Autodesk Inventor part; units mm, degrees
ref_plane "YZ Plane" through (0, 0, 0) normal (1, 0, 0) x (0, 1, 0)
ref_plane "XZ Plane" through (0, 0, 0) normal (0, 1, 0) x (-1, 0, 0)
ref_plane "XY Plane" through (0, 0, 0) normal (0, 0, 1) x (1, 0, 0)
sketch "Sketch1" plane through (0, 0, 0) normal (0, 0, 1) x (1, 0, 0)
  line L0 (20.2828, 57.747) -> (62.7008, 57.747)
  line L1 (62.7008, 57.747) -> (62.7008, 15.329)
  line L2 (62.7008, 15.329) -> (20.2828, 15.329)
  line L3 (20.2828, 15.329) -> (20.2828, 57.747)
  dimension "d0" = 42.418
  dimension "d1" = 42.418
extrude "Extrusion1" add sketch "Sketch1" along normal blind 48.006
sketch "Sketch2" plane through (0, 0, 48.006) normal (0, 0, 1) x (1, 0, 0)
  line L0 (20.2828, 57.747) -> (62.7008, 57.747)
  line L1 (20.2828, 15.329) -> (20.2828, 57.747)
  circle A0 centre (25.9978, 52.032) radius 1.5
  dimension "d4" = 3
  dimension "d5" = 5.715
  dimension "d6" = 5.715
hole "Hole1" at (25.9978, 52.032, 48.006) direction (0, 0, -1) diameter 2.4638 depth 4.5 tip angle 118
pattern_linear "Rectangular Pattern1" count 2 spacing 30.988 along (1, 0, 0) count 2 spacing 30.988 along (0, -1, 0) of "Hole1"
sketch "Sketch3" plane through (0, 0, 48.006) normal (0, 0, 1) x (1, 0, 0)
  circle A0 centre (41.4918, 36.538) radius 11.049
  dimension "d20" = 22.098
extrude "Extrusion2" add sketch "Sketch3" along normal blind 2
sketch "Sketch4" plane through (41.4918, 36.538, 50.006) normal (0, 0, 1) x (1, 0, 0)
  circle A0 centre (0, 0) radius 11.049
  circle A1 centre (0, 0) radius 2.5
  dimension "d23" = 5
extrude "Extrusion3" add sketch "Sketch4" along normal blind 22 contours A1
chamfer "Chamfer1" distance 7 angle 45 4 edges at (62.7008, 57.747, 24.003) (20.2828, 57.747, 24.003) (20.2828, 15.329, 24.003) (62.7008, 15.329, 24.003)
sketch "Sketch5" plane through (0, 0, 0) normal (0, 0, -1) x (-1, 0, 0)
  line L0 (-27.2828, 57.747) -> (-55.7008, 57.747)
  line L1 (-62.7008, 50.747) -> (-62.7008, 22.329)
  circle A0 centre (-41.4918, 36.538) radius 2.5
  dimension "d29" = 5
  dimension "d30" = 21.209
  dimension "d31" = 21.209
extrude "Extrusion4" add sketch "Sketch5" along normal blind 10
properties part number "SM-E01" material "Aluminum-6061"
Input: part model. Units: mm. Frame: model coordinates. A direction names the side the tool comes from. Coordinates: 2 decimals unless noted, no trailing zeros. Loops run counter-clockwise (first coordinate to the right, second up) from the corner with the lowest first, then second, coordinate; pieces in that order, holes last. Notation, with made-up numbers: (50.5, -4.5) -> (91.5, -4.5) arc R28 ccw to (91.5, 19.5) -> close; hole circle Ø2 at (63, 21.25). An arc over 180 degrees is marked (long way). Write each question's results on one line, items separated by ' | '. Start each with the question number.
Q1. Section B-B, the plane x = 34. Return the cut outline in (y, z).
Q2. Section C-C, the plane z = 45.5. Return the cut outline in (x, y).
Q3. Ray query, line 1 (Y direction, x = 57, z = 44); line 2 (Z direction, x = 59, y = 36); line 3 (Z direction, x = 49, y = 30). Return the intervals inside material, ascending. Write a range as from..to.
Q4. Reachability of faces 1 (the flat face through (32, 46, 48.006)), 2 (the cylindrical face through (39.182, 37.496, -4.93)), 3 (the flat face through (23.83, 18.78, 24.34)) from +Z, -Z, +X, -X, +Y, -Y: full face, straight path, thin tool, end or side. Return the list, or none.
Q5. Section D-D, the plane y = 35.5. Return the cut outline in (x, z), plus the area to 3 significant figures.
Q6. Pin query (flat end, axial travel): pin 1 (12 mm diameter, centred on x = 30.5, y = 28, fed in from +Z); pin 2 (3 mm diameter, centred on x = 56.99, y = 21.04, fed in from -Z); pin 3 (6 mm diameter, centred on x = 25.5, y = 22.5, fed in from +Z). Return the tip coordinate at first contact, or that it passes through.
Q7. Pull-direction query (X, two-part tool) for faces 4 (the conical face through (26.178, 20.929, 42.894)), 5 (the flat face through (23.734, 54.198, 24.339)), 6 (the flat face through (62.701, 37, 24)); classes: released by +X, released by -X, zero draft, split by the parting line, or undercut.
Q8. Section A-A, the plane z = 15.5. Return the cut outline in (x, y), plus the area to 3 significant figures.
Found:
1) outline: (15.33, 0) -> (57.75, 0) -> (57.75, 48.01) -> (44.66, 48.01) -> (44.66, 50.01) -> (28.42, 50.01) -> (28.42, 48.01) -> (15.33, 48.01) -> close
2) outline: (20.28, 22.33) -> (27.28, 15.33) -> (55.7, 15.33) -> (62.7, 22.33) -> (62.7, 50.75) -> (55.7, 57.75) -> (27.28, 57.75) -> (20.28, 50.75) -> close; hole circle Ø2.46 at (26, 21.04); hole circle Ø2.46 at (26, 52.03); hole circle Ø2.46 at (56.99, 21.04); hole circle Ø2.46 at (56.99, 52.03)
3) line 1: 16.63..19.81, 22.28..50.8, 53.26..56.45 | line 2: 0..48.01 | line 3: 0..50.01
4) face 1: +Z | face 2: -Z | face 3: +Z, -Z, -X, -Y
5) outline: (20.28, 0) -> (39.22, 0) -> (39.22, -10) -> (43.77, -10) -> (43.77, 0) -> (62.7, 0) -> (62.7, 48.01) -> (52.49, 48.01) -> (52.49, 50.01) -> (43.77, 50.01) -> (43.77, 72.01) -> (39.22, 72.01) -> (39.22, 50.01) -> (30.49, 50.01) -> (30.49, 48.01) -> (20.28, 48.01) -> close | area: 2,230 mm2
6) pin 1: z = 50.01 | pin 2: z = 0 | pin 3: z = 48.01
7) face 4: undercut | face 5: released by -X | face 6: released by +X
8) outline: (20.28, 22.33) -> (27.28, 15.33) -> (55.7, 15.33) -> (62.7, 22.33) -> (62.7, 50.75) -> (55.7, 57.75) -> (27.28, 57.75) -> (20.28, 50.75) -> close | area: 1,700 mm2
